Here's how the part is built. I have some questions about the finished solid (model axes, mm). A direction names the side the tool comes from. Give positions to 0.01 mm unless a question says otherwise; leave off trailing zeros. Loops run counter-clockwise (first coordinate to the right, second up) from the corner with the lowest first, then second, coordinate; pieces in that order, holes last. Notation, with made-up numbers: (58.25, -5) - (100.25, -5) arc R33 ccw to (100.25, 25) - close; hole circle Ø4 at (-16, -26). An arc over 180 degrees is marked (long way). Return JSON: item names as keys, results as strings. Group by question number.
(1) On a 3-axis mill with a long thin cutter (end or side, diameter ignored), from which of +Z, -Z, +X, -X, +Y, -Y can I reach the whole of each face in a straight line? I mean faces 4 (the flat face through (-77, 7, -24)), 5 (the flat face through (-1, 5, -45)). Say none if no direction works.
(2) I need wall thicknesses on probe 1 along X at (y, z) = (6.75, -19); probe 2 along Z at (x, y) = (-59.5, 9.75); probe 3 along X at (y, z) = (3.25, -19). Which ranges of each line are inside material? Lowest first, please. Write a range as [from, to].
(3) If we section it at B-B (x = -67): Please give me the cut outline in (y, z), then the cut area to 3 significant figures.
(4) For P1, Ø8, axis at x = -64.5, z = 23.5, coming from the +Y side, with a flat end and sliding along its axis, tell me the tip position at first contact or that it passes through.
(5) If we mould it in two halves opening along X, with no side actions, what happens to faces 1 (the flat face through (-1, 5, 45)), 2 (the flat face through (-58, 7, 24)), 3 (the flat face through (-87.5, 5, 1))? For each: released by +X, released by -X, zero draft, split by the parting line, or undercut.
(6) If we section it at A-A (y = 8.5): Please give me the cut outline in (x, z), then the cut area to 3 significant figures.
```python
from build123d import *

# Parameters (mm, degrees)
SKETCH1_W           = 175
SKETCH1_H           = 90
BOSS_EXTRUDE1_DEPTH = 10
SKETCH2_W           = 19
SKETCH2_H           = 10.1
CUT_EXTRUDE1_DEPTH  = 5.4
SKETCH2_8_R         = 1.5
CUT_EXTRUDE3_DEPTH  = 11
FILLET1_R           = 1


with BuildPart() as part:
    # Sketch1 → Boss-Extrude1 (new body)
    with BuildSketch(Plane(origin=(0, 0, 0), x_dir=(1, 0, 0), z_dir=(0, 1, 0))):
        Rectangle(SKETCH1_W, SKETCH1_H)
    extrude(amount=BOSS_EXTRUDE1_DEPTH)

    # Sketch2 → Cut-Extrude1 (cut)
    with BuildSketch(Plane(origin=(0, 10, 0), x_dir=(1, 0, 0), z_dir=(0, 1, 0))):
        with Locations((-67.5, -23.5)):
            Rectangle(SKETCH2_W, SKETCH2_H)
    cut_extrude1 = extrude(amount=-CUT_EXTRUDE1_DEPTH, mode=Mode.SUBTRACT)

    # Mirror1: Cut-Extrude1 across plane
    add(cut_extrude1.mirror(Plane.XY), mode=Mode.SUBTRACT)

    # Sketch2<8> → Cut-Extrude3 (cut, through all)
    with BuildSketch(Plane(origin=(0, 10, 0), x_dir=(1, 0, 0), z_dir=(0, 1, 0))):
        with Locations((-5, 19)):
            Circle(SKETCH2_8_R)
        with Locations((70, 19)):
            Circle(SKETCH2_8_R)
    extrude(amount=-CUT_EXTRUDE3_DEPTH, mode=Mode.SUBTRACT)

    # Fillet1
    fillet1_edges = [part.edges().sort_by_distance(p)[0] for p in [
        (-87.5, 5, -45),
        (87.5, 5, -45),
        (87.5, 5, 45),
        (-87.5, 5, 45),
    ]]
    fillet(fillet1_edges, radius=FILLET1_R)


solid = part.part
```
Values:
{
 "1": {"face 4": "+Y", "face 5": "-Z, +X, -X, +Y, -Y"},
 "2": {"probe 1": "[-87.5, -77], [-58, -6.5], [-3.5, 68.5], [71.5, 87.5]", "probe 2": "[-45, -28.55], [-18.45, 18.45], [28.55, 45]", "probe 3": "[-87.5, -6.5], [-3.5, 68.5], [71.5, 87.5]"},
 "3": {"outline": "(0, -45) - (10, -45) - (10, -28.55) - (4.6, -28.55) - (4.6, -18.45) - (10, -18.45) - (10, 18.45) - (4.6, 18.45) - (4.6, 28.55) - (10, 28.55) - (10, 45) - (0, 45) - close", "area": "791 mm2"},
 "4": {"P1": "y = 4.6"},
 "5": {"face 1": "zero draft", "face 2": "undercut", "face 3": "released by -X"},
 "6": {"outline": "(-87.5, -44) arc R1 ccw to (-86.5, -45) - (86.5, -45) arc R1 ccw to (87.5, -44) - (87.5, 44) arc R1 ccw to (86.5, 45) - (-86.5, 45) arc R1 ccw to (-87.5, 44) - close; hole (-77, -28.55) - (-58, -28.55) - (-58, -18.45) - (-77, -18.45) - close; hole (-77, 18.45) - (-58, 18.45) - (-58, 28.55) - (-77, 28.55) - close; hole circle Ø3 at (-5, -19); hole circle Ø3 at (70, -19)", "area": "15,400 mm2"}
}
